Could you check a few things on this model? Use its own coordinates, in mm. A direction names the side the tool comes from. Round coordinates to 2 decimals unless told otherwise and drop trailing zeros. Loops run counter-clockwise (first coordinate to the right, second up) from the corner with the lowest first, then second, coordinate; pieces in that order, holes last. Notation, with made-up numbers: (-36.75, 67.5) -> (15.25, 67.5) arc R25 cw to (15.25, 81.5) -> close; hole circle Ø8 at (-12.5, 5). An arc over 180 degrees is marked (long way). One line per item, written item: value.
```python
from build123d import *

# Parameters (mm, degrees)
SKETCH1_W           = 20
SKETCH1_H           = 20
BOSS_EXTRUDE1_DEPTH = 250
SKETCH2_W           = 20
SKETCH2_H           = 300
SKETCH2_W_2         = 300
SKETCH2_H_2         = 20
BOSS_EXTRUDE2_DEPTH = 10


with BuildPart() as part:
    # Sketch1 → Boss-Extrude1 (new body)
    with BuildSketch(Plane(origin=(0, 0, 0), x_dir=(1, 0, 0), z_dir=(0, 1, 0))):
        Rectangle(SKETCH1_W, SKETCH1_H)
    extrude(amount=BOSS_EXTRUDE1_DEPTH)

    # Sketch2 → Boss-Extrude2 (add)
    with BuildSketch(Plane(origin=(0, 0, 0), x_dir=(1, 0, 0), z_dir=(0, 1, 0))):
        with Locations((0, -160)):
            Rectangle(SKETCH2_W, SKETCH2_H)
        with Locations((160, 0)):
            Rectangle(SKETCH2_W_2, SKETCH2_H_2)
    extrude(amount=BOSS_EXTRUDE2_DEPTH)


solid = part.part
```
Item 1: Will these pins go through, and if not, where does the flat tip stop? pin 1 Ø3 at (x, y) = (193, 3.5) entering from +Z; pin 2 Ø8 at (y, z) = (3.5, 132.5) entering from +X; pin 3 Ø6 at (x, z) = (100.5, 0.5) entering from +Y.
Output:
pin 1: stops at z = 10
pin 2: stops at x = 10
pin 3: stops at y = 10
Item 2: If we section it at B-B on z = 120.5: List the corners of the cut face in (x, y) for me.
Output:
outline: (-10, 0) -> (10, 0) -> (10, 10) -> (-10, 10) -> close
Item 3: I need wall thicknesses on line 1 (Y direction, x = 6, z = 225.5). Which ranges of the line are inside material? Lowest first, please. Write a range as from..to.
Output:
line 1: y = 0..10
Item 4: For faces 1 (the face through (0, 128, 10)), 2 (the face through (158, 10, 0)), 3 (the face through (10, 5, 162)), 4 (the face through (-10, 87, 9)), which set-ups out of +Z, -Z, +X, -X, +Y, -Y let a thin tool reach every point of the face, with its end or its side?
Output:
face 1: +Z, +X, -X, +Y
face 2: +Z, -Z, +X, +Y
face 3: +Z, +X, +Y, -Y
face 4: +Z, -Z, -X, +Y, -Y
Item 5: If we section it at A-A on x = 52.5: List the corners of the cut face in (y, z) for me.
Output:
outline: (0, -10) -> (10, -10) -> (10, 10) -> (0, 10) -> close
